Build history of the part. All positions in model axes, mm. A direction names the side the tool comes from. Give positions to 0.01 mm unless a question says otherwise; leave off trailing zeros. Loops run counter-clockwise (first coordinate to the right, second up) from the corner with the lowest first, then second, coordinate; pieces in that order, holes last. Notation, with made-up numbers: (41.5, -22.5) -> (51.5, -22.5) arc R26 ccw to (51.5, 11.5) -> close; hole circle Ø10 at (-9, 51). An arc over 180 degrees is marked (long way). Answer as a JSON object with one key per item and string values. Group by question number.
Q1. Band-saw the part on B-B, the plane x = -10. Write the cut outline in (y, z).
Q2. Tool access for faces 5 (the cylindrical face through (-0.57, 4.4, -29.58)), 6 (the flat face through (-30, 4.9, -30)): list every direction of +Z, -Z, +X, -X, +Y, -Y with a clear straight run to the whole face (end or side of a thin tool).
Q3. Band-saw the part on C-C, the plane z = -30. Write the cut outline in (x, y), plus the area to 3 significant figures.
Q4. Drop flat-ended pins along their axis: pin 1 (3.5 mm diameter, centred on x = -5, z = -5, fed in from -Y); pin 2 (10 mm diameter, centred on x = -34.5, z = -30.5, fed in from -Y); pin 3 (15 mm diameter, centred on x = -40, z = -27.5, fed in from +Y); pin 4 (5.5 mm diameter, centred on x = -5, z = -55, fed in from +Y). Give the stop position or say it passes through.
Q5. Two-plate mould, pull along X, no slides. Class faces 1 (the cylindrical face through (-59.43, 4.4, -30.42)), 2 (the cylindrical face through (-55.09, 2.05, -7.15)), 3 (the flat face through (-4.7, 5, -29.6)), 4 (the cylindrical face through (-5.09, 2.05, -57.15)): pulls with the +X half, pulls with the -X half, needs draft (parallel to the pull), parting line crosses it, or undercut.
Q6. Wall check: probe 1 along Z at (x, y) = (-55, 1.65); probe 2 along Y at (x, z) = (-30, -44). Give the ranges that are in metal, low to high. Write a range as from..to.
Q7. Band-saw the part on A-A, the plane y = 2.2. Write the cut outline in (x, z).
Q8. Band-saw the part on D-D, the plane x = -4. Count the separate pieces of the cut face and the enclosed holes in it, plus the area to 3 significant figures.
Autodesk Inventor part; units mm, degrees
ref_plane "YZ Plane" through (0, 0, 0) normal (1, 0, 0) x (0, 1, 0)
ref_plane "XZ Plane" through (0, 0, 0) normal (0, 1, 0) x (-1, 0, 0)
ref_plane "XY Plane" through (0, 0, 0) normal (0, 0, 1) x (1, 0, 0)
sketch "Sketch1" plane through (0, 0, 0) normal (0, 1, 0) x (-1, 0, 0)
  line L0 (0, 0) -> (60, 0)
  line L1 (60, 0) -> (60, -60)
  line L2 (60, -60) -> (0, -60)
  line L3 (0, -60) -> (0, 0)
  dimension "d0" = 60
  dimension "d1" = 60
extrude "Extrusion1" add sketch "Sketch1" along normal blind 5
sketch "Sketch2" plane through (0, 5, 0) normal (0, 1, 0) x (1, 0, 0)
  line L0 (-60, 0) -> (0, 0)
  line L1 (0, 0) -> (0, 60)
  line L2 (0, 60) -> (-60, 60)
  line L3 (-60, 60) -> (-60, 0)
  point P0 (-5, 5)
  point P1 (-5, 55)
  point P2 (-55, 55)
  point P3 (-55, 5)
  dimension "d4" = 5
  dimension "d6" = 5
  dimension "d7" = 5
  dimension "d8" = 5
  dimension "d9" = 5
  dimension "d10" = 5
  dimension "d11" = 5
  dimension "d12" = 5
hole "Hole1" at (-5, 5, -5) at (-5, 5, -55) at (-55, 5, -55) at (-55, 5, -5) direction (0, -1, 0) diameter 4.3 end through all countersink diameter 6 countersink angle 90
fillet "Fillet1" radius 2 4 edges at (-30, 5, 0) (-60, 5, -30) (-30, 5, -60) (0, 5, -30)
sketch "Sketch3" plane through (0, 5, 0) normal (0, 1, 0) x (1, 0, 0)
  circle A0 centre (-30, 30) radius 25
  line L0 (-60, 0) -> (0, 0)
  line L1 (-60, 60) -> (-60, 0)
  dimension "d21" = 30
  dimension "d22" = 30
  dimension "d23" = 50
extrude "Extrusion2" cut sketch "Sketch3" against normal blind 0.1
properties part number "Filter"
Worked answers:
{
 "1": {"outline": "(0, -60) -> (3, -60) arc R2 ccw to (5, -58) -> (5, -45) -> (4.9, -45) -> (4.9, -15) -> (5, -15) -> (5, -2) arc R2 ccw to (3, 0) -> (0, 0) -> close"},
 "2": {"face 5": "+Z, -Z, +X, +Y", "face 6": "+Y"},
 "3": {"outline": "(-60, 0) -> (0, 0) -> (0, 3) arc R2 ccw to (-2, 5) -> (-5, 5) -> (-5, 4.9) -> (-55, 4.9) -> (-55, 5) -> (-58, 5) arc R2 ccw to (-60, 3) -> close", "area": "293 mm2"},
 "4": {"pin 1": "through", "pin 2": "y = 0", "pin 3": "y = 4.9", "pin 4": "y = 4.75"},
 "5": {"face 1": "pulls with the -X half", "face 2": "undercut", "face 3": "needs draft", "face 4": "undercut"},
 "6": {"probe 1": "-60..-57.15, -52.85..-7.15, -2.85..0", "probe 2": "0..4.9"},
 "7": {"outline": "(-60, -60) -> (0, -60) -> (0, 0) -> (-60, 0) -> close; hole circle Ø4.3 at (-55, -55); hole circle Ø4.3 at (-55, -5); hole circle Ø4.3 at (-5, -55); hole circle Ø4.3 at (-5, -5)"},
 "8": {"separate pieces": "3", "enclosed holes": "0", "area": "259 mm2"}
}
